```python
from build123d import *

# Parameters (mm, degrees)
SKETCH1_R               = 7
SKETCH1_R_2             = 4
BOSS_EXTRUDE1_DEPTH     = 25
BOSS_EXTRUDE2_START     = -12.5
SKETCH2_R               = 4
SKETCH2_R_2             = 2.5
BOSS_EXTRUDE2_DEPTH     = 12.5
CUT_EXTRUDE1_DEPTH      = 27.888659319
CUT_EXTRUDE1_DEPTH_BACK = 27.888659319
SKETCH3_R               = 2


with BuildPart() as part:
    # Sketch1 → Boss-Extrude1 (new body)
    with BuildSketch(Plane.XY):
        Circle(SKETCH1_R)
        Circle(SKETCH1_R_2, mode=Mode.SUBTRACT)
    extrude(amount=BOSS_EXTRUDE1_DEPTH)

    # Sketch2 → Boss-Extrude2 (add)
    with BuildSketch(Plane.XY.offset(25).offset(BOSS_EXTRUDE2_START)):
        Circle(SKETCH2_R)
        Circle(SKETCH2_R_2, mode=Mode.SUBTRACT)
    extrude(amount=BOSS_EXTRUDE2_DEPTH)

    # Sketch3 → Cut-Extrude1 (cut, two sides: drawn at the far end of the back side and taken through both)
    with BuildSketch(Plane(origin=(0, 0, 0), x_dir=(1, 0, 0), z_dir=(0, 1, 0)).offset(-CUT_EXTRUDE1_DEPTH_BACK)):
        with Locations(Location((0, -7.5, 0), (0, 0, 270))):
            Circle(SKETCH3_R)
        with Locations(Location((0, -17.5, 0), (0, 0, 270))):
            Circle(SKETCH3_R)
    extrude(amount=CUT_EXTRUDE1_DEPTH + CUT_EXTRUDE1_DEPTH_BACK, mode=Mode.SUBTRACT)


solid = part.part
```
Verification items for the finished model (mm, model axes). A direction names the side the tool comes from. Give positions to 0.01 mm unless a question says otherwise; leave off trailing zeros. Loops run counter-clockwise (first coordinate to the right, second up) from the corner with the lowest first, then second, coordinate; pieces in that order, holes last. Notation, with made-up numbers: M 29,-28.75 L 87,-28.75 A30 cw 87,-6.75 Z; hole C 13.5,16 d3. An arc over 180 degrees is marked long. Return JSON: item names as keys, results as strings.
1) Section check D-D, the plane z = 14. Enter the section's corners in (x, y), and give its area (3 significant figures).
Findings:
{"outline": "C 0,0 d14; hole C 0,0 d5", "area": "134 mm2"}
2) Section check C-C, the plane z = 6.75. Enter the section's corners in (x, y).
Findings:
{"outline": "M -1.85,-6.75 L -1.85,-3.54 A4 cw -1.85,3.54 L -1.85,6.75 A7 ccw Z; M 1.85,-6.75 A7 ccw 1.85,6.75 L 1.85,3.54 A4 cw 1.85,-3.54 Z"}
3) Tool access check on faces 1 (the cylindrical face through (-0.766, -4.292, 19.347)), 2 (the cylindrical face through (2.15, 3.373, 6.162)). Record the directions out of +Z, -Z, +X, -X, +Y, -Y that give a thin tool (end or side, any length) a straight path to the whole face; none if there is none.
Findings:
{"face 1": "+Y, -Y", "face 2": "-Z"}
4) Section check A-A, the plane x = 0. Enter the section's corners in (y, z).
Findings:
{"outline": "M -7,0 L -4,0 L -4,5.5 L -7,5.5 Z; M -7,9.5 L -4,9.5 L -4,12.5 L -2.5,12.5 L -2.5,15.5 L -7,15.5 Z; M -7,19.5 L -2.5,19.5 L -2.5,25 L -7,25 Z; M 2.5,12.5 L 4,12.5 L 4,9.5 L 7,9.5 L 7,15.5 L 2.5,15.5 Z; M 2.5,19.5 L 7,19.5 L 7,25 L 2.5,25 Z; M 4,0 L 7,0 L 7,5.5 L 4,5.5 Z"}
5) Mould release check, pull along Z, two halves, no side actions. Record for faces 3 (the cylindrical face through (-1.2, 4.2, 15.9)), 4 (the cylindrical face through (-1.2, -5.3, 5.9)), 5 (the flat face through (2, 2, 12.5)), 6 (the flat face through (0, -3, 25)): released by +Z, released by -Z, zero draft, split by the parting line, or undercut.
Findings:
{"face 3": "undercut", "face 4": "undercut", "face 5": "released by -Z", "face 6": "released by +Z"}
6) Gauge pin test, flat ends, axial feed: P1, Ø1, axis at x = -3, z = 20.5, coming from the +Y side; P2, Ø2, axis at x = -2.5, z = 14.5, coming from the +Y side; P3, Ø4, axis at x = -2.5, z = 11.5, coming from the -Y side. Record the tip position at first contact, or that the pin passes through.
Findings:
{"P1": "stops at y = 6.54", "P2": "stops at y = 6.84", "P3": "stops at y = -6.98"}
7) Material ranges on L1, parallel to Z at x = 0, y = -4.75; L2, parallel to X at y = -2, z = 3.5; L3, parallel to X at y = -1.75, z = 6.25, recorded low to high. Write a range as [from, to].
Findings:
{"L1": "z = [0, 5.5], [9.5, 15.5], [19.5, 25]", "L2": "x = [-6.71, -3.46], [3.46, 6.71]", "L3": "x = [-6.78, -3.6], [3.6, 6.78]"}
8) Section check B-B, the plane y = 0. Enter the section's corners in (x, z), and give its area (4 significant figures).
Findings:
{"outline": "M -7,0 L -4,0 L -4,12.5 L -2.5,12.5 L -2.5,25 L -7,25 Z; M 2.5,12.5 L 4,12.5 L 4,0 L 7,0 L 7,25 L 2.5,25 Z", "area": "187.5 mm2"}
